```python
from build123d import *

# Parameters (mm, degrees)
SKETCH1_W             = 47.7
SKETCH1_H             = 45.7
BOSS_EXTRUDE1_DEPTH   = 1.5
SKETCH2_W             = 47.7
SKETCH2_H             = 3
BOSS_EXTRUDE2_DEPTH   = 4
SKETCH3_W             = 47.7
SKETCH3_H             = 3
CUT_EXTRUDE1_DEPTH    = 1.2
SKETCH4_W             = 47.7
SKETCH4_H             = 3
CUT_EXTRUDE2_DEPTH    = 1.2
SKETCH5_R             = 1.5
CUT_EXTRUDE3_DEPTH    = 67.179906316
SKETCH8_W             = 39.7
SKETCH8_H             = 4
CUT_EXTRUDE5_DEPTH    = 63.494319742
SKETCH9_W             = 18.85
SKETCH9_H             = 5.7
CUT_EXTRUDE6_DEPTH    = 67.179906316
FILLET1_R             = 2
BODY_MOVE_COPY1_ANGLE = 90


with BuildPart() as part:
    # Sketch1 → Boss-Extrude1 (new body)
    with BuildSketch(Plane(origin=(0, 0, 0), x_dir=(1, 0, 0), z_dir=(0, 1, 0))):
        with Locations((23.85, 22.85)):
            Rectangle(SKETCH1_W, SKETCH1_H)
    extrude(amount=BOSS_EXTRUDE1_DEPTH)

    # Sketch2 → Boss-Extrude2 (add)
    with BuildSketch(Plane(origin=(0, 1.5, 0), x_dir=(1, 0, 0), z_dir=(0, 1, 0))):
        with Locations((23.85, 38.5)):
            Rectangle(SKETCH2_W, SKETCH2_H)
        with Locations((23.85, 7.2)):
            Rectangle(SKETCH2_W, SKETCH2_H)
    extrude(amount=BOSS_EXTRUDE2_DEPTH)

    # Sketch3 → Cut-Extrude1 (cut)
    with BuildSketch(Plane.XY.offset(-37)):
        with Locations((23.85, 3)):
            Rectangle(SKETCH3_W, SKETCH3_H)
    extrude(amount=-CUT_EXTRUDE1_DEPTH, mode=Mode.SUBTRACT)

    # Sketch4 → Cut-Extrude2 (cut)
    with BuildSketch(Plane(origin=(0, 0, -8.7), x_dir=(-1, 0, 0), z_dir=(0, 0, -1))):
        with Locations((-23.85, 3)):
            Rectangle(SKETCH4_W, SKETCH4_H)
    extrude(amount=-CUT_EXTRUDE2_DEPTH, mode=Mode.SUBTRACT)

    # Sketch5 → Cut-Extrude3 (cut, through all)
    with BuildSketch(Plane(origin=(0, 1.5, 0), x_dir=(1, 0, 0), z_dir=(0, 1, 0))):
        with Locations(Location((23.85, 42.85, 0), (0, 0, 270))):
            Circle(SKETCH5_R)
        with Locations(Location((23.85, 2.85, 0), (0, 0, 270))):
            Circle(SKETCH5_R)
    extrude(amount=-CUT_EXTRUDE3_DEPTH, mode=Mode.SUBTRACT)

    # Sketch8 → Cut-Extrude5 (cut, through all)
    with BuildSketch(Plane.XY.offset(-5.7)):
        with Locations((23.85, 3.5)):
            Rectangle(SKETCH8_W, SKETCH8_H)
    extrude(amount=-CUT_EXTRUDE5_DEPTH, mode=Mode.SUBTRACT)

    # Sketch9 → Cut-Extrude6 (cut, through all)
    with BuildSketch(Plane(origin=(0, 1.5, 0), x_dir=(1, 0, 0), z_dir=(0, 1, 0))):
        with Locations((9.425, 42.85)):
            Rectangle(SKETCH9_W, SKETCH9_H)
        with Locations((38.275, 42.85)):
            Rectangle(SKETCH9_W, SKETCH9_H)
        with Locations((38.275, 2.85)):
            Rectangle(SKETCH9_W, SKETCH9_H)
        with Locations((9.425, 2.85)):
            Rectangle(SKETCH9_W, SKETCH9_H)
    extrude(amount=-CUT_EXTRUDE6_DEPTH, mode=Mode.SUBTRACT)

    # Fillet1
    fillet1_edges = [part.edges().sort_by_distance(p)[0] for p in [
        (18.85, 0.75, 0),
        (18.85, 0.75, -5.7),
        (28.85, 0.75, 0),
        (28.85, 0.75, -5.7),
        (28.85, 0.75, -45.7),
        (28.85, 0.75, -40),
        (18.85, 0.75, -45.7),
        (18.85, 0.75, -40),
    ]]
    fillet(fillet1_edges, radius=FILLET1_R)


with BuildPart() as part_1:
    # Body-Move/Copy1: moved
    add(part.part.rotate(Axis((0, 2.75, -20.7), (1, 0, 0)), BODY_MOVE_COPY1_ANGLE))


solid = part_1.part
```
Read the model definition and answer for the solid it produces. Units are mm, in the model's axes. A direction names the side the tool comes from. Give positions to 0.01 mm unless a question says otherwise; leave off trailing zeros. Order: outer loops, then holes, each group sorted by start corner. A loop starts at its lowest first (then second) coordinate and runs counter-clockwise, first axis right, second up.
(1) Straight lines are drawn through the part: L1, parallel to X at y = -15.1, z = -22.3; L2, parallel to X at y = -11, z = -21; L3, parallel to Z at x = 16, y = 14. For each, find the intervals that lie inside material, in ascending order.
(2) Given pin 1 (0.9 mm diameter, centred on x = 2, z = -20.5, fed in from +Y); pin 2 (0.5 mm diameter, centred on x = 45, z = -18.5, fed in from -Y); pin 3 (4 mm diameter, centred on x = 23.85, y = 24.9, fed in from +Z), each flat-ended and moving along its own axis, determine where each tip first touches the part or whether it passes through.
(3) Find section A-A (x = 23.85). Give the vertices of the cut face in (y, z).
(4) For faces 4 (the flat face through (18.85, -15, -23)), 5 (the flat face through (2, -9.25, -18.5)), 6 (the flat face through (46, -10.45, -20)), determine the directions among +Z, -Z, +X, -X, +Y, -Y from which every point of the face is accessible in a straight line to the end or side of a thin tool.
(5) For a pull along X with two mould halves and no side action, classify faces 1 (the cylindrical face through (24.86, 26.01, -22.69)), 2 (the flat face through (2, -10, -18.95)), 3 (the cylindrical face through (28.25, 27.18, -22.71)) as released by +X, released by -X, zero draft, split by the parting line, or undercut.
(6) Find section D-D (y = -15.1). Give the vertices of the cut face in (x, z), plus the area to 3 significant figures.
(7) Find section C-C (y = 21). Give the vertices of the cut face in (x, z), plus the area to 3 significant figures.
(8) Find section B-B (z = -20.9). Give the vertices of the cut face in (x, y).
Result sheet:
1. L1: x = 18.85 to 22.35, 25.35 to 28.85
1. L2: x = 0 to 4, 43.7 to 47.7
1. L3: z = -23.45 to -21.95
2. pin 1: stops at y = 22.05
2. pin 2: stops at y = -12.25
2. pin 3: stops at z = -21.95
3. outline: (-17.95, -23.45) - (-16.6, -23.45) - (-16.6, -21.95) - (-17.95, -21.95) - close; (-13.6, -23.45) - (23.4, -23.45) - (23.4, -21.95) - (-13.6, -21.95) - close; (26.4, -23.45) - (27.75, -23.45) - (27.75, -21.95) - (26.4, -21.95) - close
4. face 4: +Z, -Z, -X, -Y
4. face 5: +Z, +X, -X
4. face 6: +X, -X
5. face 1: undercut
5. face 2: zero draft
5. face 3: released by +X
6. outline: (18.85, -23.45) - (22.35, -23.45) - (22.35, -21.95) - (18.85, -21.95) - close; (25.35, -23.45) - (28.85, -23.45) - (28.85, -21.95) - (25.35, -21.95) - close
6. area: 10.5 mm2
7. outline: (0, -23.45) - (47.7, -23.45) - (47.7, -17.95) - (43.7, -17.95) - (43.7, -21.95) - (4, -21.95) - (4, -17.95) - (0, -17.95) - close
7. area: 104 mm2
8. outline: (0, -12.25) - (4, -12.25) - (4, -10.45) - (0, -10.45) - close; (0, 20.25) - (4, 20.25) - (4, 22.05) - (0, 22.05) - close; (43.7, -12.25) - (47.7, -12.25) - (47.7, -10.45) - (43.7, -10.45) - close; (43.7, 20.25) - (47.7, 20.25) - (47.7, 22.05) - (43.7, 22.05) - close
